from build123d import *

# Parameters (mm, degrees)
F0_R     = 2
F1_DEPTH = 100
F2_R     = 2.5
F3_DEPTH = 10
F4_R     = 2.5
F5_W     = 0.722433
F5_H     = 5.884245
F5_W_2   = 2
F5_W_3   = 0.957619
F6_DEPTH = 3.08
F7_R     = 1
F8_DEPTH = 4.501


with BuildPart() as f1:
    # F0 (on Top) → F1 (new body)
    with BuildSketch(Plane.XY):
        Circle(F0_R)
    extrude(amount=F1_DEPTH)

    # F2 (on face) → F3 (join)
    with BuildSketch(Plane(origin=(0, 0, 0), x_dir=(1, 0, 0), z_dir=(0, 0, -1))):
        Circle(F2_R)
    extrude(amount=F3_DEPTH)

    # F4
    f4_edges = [f1.edges().sort_by_distance(p)[0] for p in [
        (-2.5, 0, -10),
    ]]
    fillet(f4_edges, radius=F4_R)

    # F5 (on Front) → F6 (cut, symmetric)
    with BuildSketch(Plane.XZ):
        with Locations((-2.361216, -7.442122)):
            Rectangle(F5_W, F5_H)
        with Locations((0, -7.442122)):
            Rectangle(F5_W_2, F5_H)
        with Locations((2.478809, -7.442122)):
            Rectangle(F5_W_3, F5_H)
    extrude(amount=F6_DEPTH, both=True, mode=Mode.SUBTRACT)

    # F7 (on face) → F8 (cut, through all)
    with BuildSketch(Plane(origin=(-2, 0, 0), x_dir=(0, -1, 0), z_dir=(-1, 0, 0))):
        with Locations((0, -7.5)):
            Circle(F7_R)
    extrude(amount=-F8_DEPTH, mode=Mode.SUBTRACT)


solid = f1.part
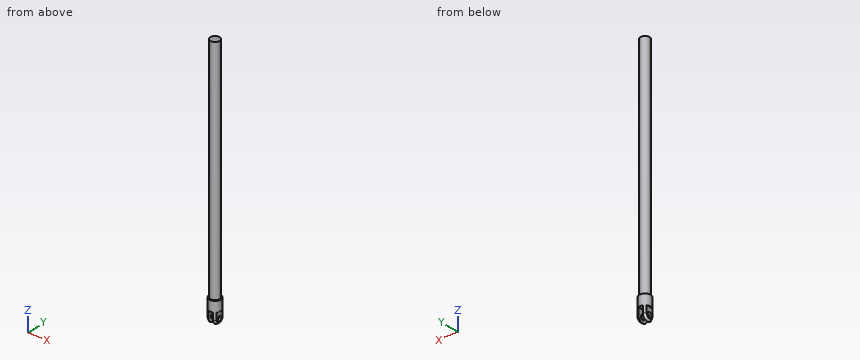
The listing builds one solid part. Answer for the finished solid, in the listing's coordinates (mm). Coordinates: 2 decimals unless noted, no trailing zeros. Write each loop counter-clockwise with the first axis right and the second up, starting at its lowest first coordinate (ties: lowest second). Pieces come first, ordered by that corner, then holes. Notation, with made-up numbers: M 6.5,70 L 52.5,70 A14 cw 52.5,86 Z; hole C -0.5,0 d6. An arc over 180 degrees is marked long. Put each result on its own line as item: value. Start each with the question number.
1. Consider line 1 (Z direction, x = -0.45, y = -1.25); line 2 (X direction, y = 0.05, z = 26.5); line 3 (Z direction, x = -1.4, y = 0). Determine where each line is inside the solid, lowest interval first. Write a range as from..to.
2. Flat-ended cylindrical pins translate along their axes: P1, Ø0.6, axis at x = 2, y = -0.5, coming from the -Z side; P2, Ø1, axis at y = -1.5, z = 37.5, coming from the -X side; P3, Ø2.5, axis at y = 0, z = -7.5, coming from the -X side. Find the tip coordinate at first contact, or state that the pin passes through.
3. A cutting plane is placed at C-C on z = 80. Write down the section's boundary in (x, y).
4. A cutting plane is placed at A-A on y = 0. Write down the section's boundary in (x, z).
5. A cutting plane is placed at B-B on x = 0. Write down the section's boundary in (y, z), then the cut area to 4 significant figures.
Resolved:
1. line 1: z = -4.5..100
1. line 2: x = -2..2
1. line 3: z = -9.57..-8.5, -6.5..100
2. P1: stops at z = -9.27
2. P2: stops at x = -1.73
2. P3: stops at x = -2
3. outline: C 0,0 d4
4. outline: M -2.5,-4.5 L -2,-4.5 L -2,-6.5 L -1,-6.5 L -1,-4.5 L 1,-4.5 L 1,-6.5 L 2,-6.5 L 2,-4.5 L 2.5,-4.5 L 2.5,0 L 2,0 L 2,100 L -2,100 L -2,0 L -2.5,0 Z; M -2,-9 A2.5 ccw -1,-9.79 L -1,-8.5 L -2,-8.5 Z; M 1,-9.79 A2.5 ccw 2,-9 L 2,-8.5 L 1,-8.5 Z
5. outline: M -2.5,-4.5 L 2.5,-4.5 L 2.5,0 L 2,0 L 2,100 L -2,100 L -2,0 L -2.5,0 Z
5. area: 422.5 mm2
